Solid Edge part; units mm, degrees
sketch "Sketch1" plane through (0, 0, 0) normal (0, -1, 0) x (1, 0, 0)
  line L0 (22.5, -27.5) -> (22.5, 27.5)
  line L1 (22.5, 27.5) -> (-22.5, 27.5)
  line L2 (-22.5, 27.5) -> (-22.5, -27.5)
  line L3 (-22.5, -27.5) -> (22.5, -27.5)
extrude "Protrusion1" add sketch "Sketch1" against normal blind 1.5
sketch "Sketch2" plane through (0, 0, 0) normal (0, -1, 0) x (1, 0, 0)
  circle A0 centre (-3.45, 14.41) radius 1.5
  circle A1 centre (-7.9, -11) radius 1.5
extrude "ExtrudedCutout_1" cut sketch "Sketch2" against normal blind 1.7648
sketch "Sketch3" plane through (0, 0, 0) normal (0, -1, 0) x (1, 0, 0)
  line L0 (-10.1147, 15.2675) -> (-20.4202, 15.2675)
  line L1 (-20.4202, 15.2675) -> (-20.4202, 25.6684)
  line L2 (-20.4202, 25.6684) -> (-10.1147, 25.6684)
  line L3 (-10.1147, 25.6684) -> (-10.1147, 15.2675)
  line L4 (-13.6, 5.8207) -> (-20.134, 5.8207)
  line L5 (-20.134, 5.8207) -> (-20.134, 12.7865)
  line L6 (-20.134, 12.7865) -> (-13.6, 12.7865)
  line L7 (-13.6, 12.7865) -> (-13.6, 5.8207)
  line L8 (-20.8019, 2.6718) -> (-10.5918, 2.6718)
  line L9 (-10.5918, 2.6718) -> (-10.5918, -8.1108)
  line L10 (-10.5918, -8.1108) -> (-20.8019, -8.1108)
  line L11 (-20.8019, -8.1108) -> (-20.8019, 2.6718)
extrude "ExtrudedProtrusion_2" add sketch "Sketch3" along normal blind 2
sketch "Sketch4" plane through (0, 0, 0) normal (0, -1, 0) x (1, 0, 0)
  line L0 (-16.7942, -24.9) -> (-20.8019, -24.9)
  line L1 (-20.8019, -24.9) -> (-20.8019, -11.546)
  line L2 (-20.8019, -11.546) -> (-16.7942, -11.546)
  line L3 (-16.7942, -11.546) -> (-16.7942, -24.9)
extrude "ExtrudedProtrusion_3" add sketch "Sketch4" along normal blind 2.5
sketch "Sketch5" plane through (0, 0, 0) normal (0, -1, 0) x (1, 0, 0)
  line L0 (-0.7713, -24.7674) -> (-0.7713, -12.8397)
  line L1 (-0.7713, -12.8397) -> (5.2403, -12.8397)
  line L2 (5.2403, -12.8397) -> (5.2403, -24.7674)
  line L3 (5.2403, -24.7674) -> (-0.7713, -24.7674)
extrude "ExtrudedProtrusion_6" add sketch "Sketch5" along normal blind 2
sketch "Sketch6" plane through (0, 0, 0) normal (0, -1, 0) x (1, 0, 0)
  line L0 (18.5118, -7.0612) -> (1.4313, -7.0612)
  line L1 (1.4313, -7.0612) -> (1.4313, 3.9123)
  line L2 (1.4313, 3.9123) -> (18.5118, 3.9123)
  line L3 (18.5118, 3.9123) -> (18.5118, -7.0612)
extrude "ExtrudedProtrusion_7" add sketch "Sketch6" along normal blind 2.5
sketch "Sketch7" plane through (0, 0, 0) normal (0, -1, 0) x (1, 0, 0)
  circle A0 centre (18.1072, 22.9106) radius 4.1
extrude "ExtrudedProtrusion_8" add sketch "Sketch7" along normal blind 12.5
sketch "Sketch8" plane through (0, 0, 0) normal (0, -1, 0) x (1, 0, 0)
  circle A0 centre (18.1928, 14.1814) radius 4.1
extrude "ExtrudedProtrusion_9" add sketch "Sketch8" along normal blind 12.5
fillet "Round_1" radius 0.5 2 edges at (14.0928, -12.5, 14.1814) (14.0072, -12.5, 22.9106)
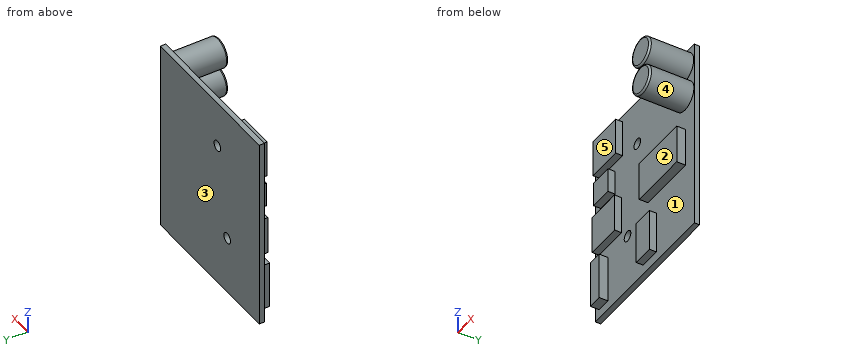
Check sheet for the modelled part. Datum: model origin and axes. Units: mm. Face numbers are marked on the shaded views. A direction names the side the tool comes from. Round coordinates to 2 decimals unless told otherwise and drop trailing zeros. Loops run counter-clockwise (first coordinate to the right, second up) from the corner with the lowest first, then second, coordinate; pieces in that order, holes last.
1. Set-up check for the marked faces 3, 4 and 5: record each of +Z, -Z, +X, -X, +Y, -Y from which the full face is reachable in a straight line by a thin tool's end or side.
2. Sectioned sample at C-C on x = -16. Record the boundary of the cut face in (y, z), and give its area (3 significant figures).
3. Sectioned sample at A-A on x = -7.9. Record the boundary of the cut face in (y, z).
4. Mould release check, pull along X, two halves, no side actions. Record for the marked faces 1 and 2: released by +X, released by -X, zero draft, split by the parting line, or undercut.
5. Sectioned sample at D-D on y = -10.5. Record the boundary of the cut face in (x, z), and give its area (3 significant figures).
6. Sectioned sample at B-B on z = -1.5. Record the boundary of the cut face in (x, y).
7. Gauge pin test, flat ends, axial feed: pin 1 Ø0.6 at (x, y) = (1.5, -0.5) entering from -Z; pin 2 Ø8 at (x, z) = (-14.5, 21) entering from -Y; pin 3 Ø1 at (y, z) = (-1, -5) entering from -X. Record the tip position at first contact, or that the pin passes through.
8. Scan lines: probe 1 along Z at (x, y) = (-7.9, 1); probe 2 along Z at (x, y) = (-3.45, 0.5); probe 3 along Y at (x, z) = (-10, 3). Record each from-to range of solid material in increasing order.
Recorded:
1. face 3: +Z, -Z, +X, -X, +Y
1. face 4: -Y
1. face 5: +Z, -X, -Y
2. outline: (-2, -8.11) - (0, -8.11) - (0, -27.5) - (1.5, -27.5) - (1.5, 27.5) - (0, 27.5) - (0, 25.67) - (-2, 25.67) - (-2, 15.27) - (0, 15.27) - (0, 12.79) - (-2, 12.79) - (-2, 5.82) - (0, 5.82) - (0, 2.67) - (-2, 2.67) - close
2. area: 139 mm2
3. outline: (0, -27.5) - (1.5, -27.5) - (1.5, -12.5) - (0, -12.5) - close; (0, -9.5) - (1.5, -9.5) - (1.5, 27.5) - (0, 27.5) - close
4. face 1: undercut
4. face 2: zero draft
5. outline: circle Ø8.2 at (18.11, 22.91); circle Ø8.2 at (18.19, 14.18)
5. area: 106 mm2
6. outline: (-22.5, 0) - (-20.8, 0) - (-20.8, -2) - (-10.59, -2) - (-10.59, 0) - (1.43, 0) - (1.43, -2.5) - (18.51, -2.5) - (18.51, 0) - (22.5, 0) - (22.5, 1.5) - (-22.5, 1.5) - close
7. pin 1: stops at z = -24.77
7. pin 2: stops at y = -2
7. pin 3: stops at x = -20.8
8. probe 1: z = -27.5 to -12.5, -9.5 to 27.5
8. probe 2: z = -27.5 to 12.91, 15.91 to 27.5
8. probe 3: y = 0 to 1.5
